from build123d import *

# Parameters (mm, degrees)
F0_W     = 3
F0_H     = 3
F1_DEPTH = 0.15
F2_DEPTH = 1.9
F3_W     = 0.15
F3_H     = 7
F4_DEPTH = 5
F6_DEPTH = 25
F7_R     = 0.5


with BuildPart() as f1:
    # F0 (on Top) → F1 (new body)
    with BuildSketch(Plane.XY):
        with Locations((72.2, 2)):
            Rectangle(F0_W, F0_H)
        with BuildLine():
            Line((10.1, -0.5), (10.1, -3.5))
            Line((10.1, -3.5), (20.2, -3.5))
            Line((20.2, -3.5), (30.3, -3.5))
            Line((30.3, -3.5), (30.3, -0.5))
            Line((30.3, -0.5), (25.7, -0.5))
            ThreePointArc((25.7, -0.5), (25.4171572875, -0.3828427125), (25.3, -0.1))
            Line((25.3, -0.1), (25.3, 0.1))
            ThreePointArc((25.3, 0.1), (25.4171572875, 0.3828427125), (25.7, 0.5))
            Line((25.7, 0.5), (30.3, 0.5))
            Line((30.3, 0.5), (30.3, 3.5))
            Line((30.3, 3.5), (20.2, 3.5))
            Line((20.2, 3.5), (10.1, 3.5))
            Line((10.1, 3.5), (10.1, 0.5))
            Line((10.1, 0.5), (14.7, 0.5))
            ThreePointArc((14.7, 0.5), (14.9828427125, 0.3828427125), (15.1, 0.1))
            Line((15.1, 0.1), (15.1, -0.1))
            ThreePointArc((15.1, -0.1), (14.9828427125, -0.3828427125), (14.7, -0.5))
            Line((14.7, -0.5), (10.1, -0.5))
        make_face()
        with BuildLine():
            Line((30.3, -0.5), (30.3, -3.5))
            Line((30.3, -3.5), (40.4, -3.5))
            Line((40.4, -3.5), (50.5, -3.5))
            Line((50.5, -3.5), (50.5, -0.5))
            Line((50.5, -0.5), (45.9, -0.5))
            ThreePointArc((45.9, -0.5), (45.6171572875, -0.3828427125), (45.5, -0.1))
            Line((45.5, -0.1), (45.5, 0.1))
            ThreePointArc((45.5, 0.1), (45.6171572875, 0.3828427125), (45.9, 0.5))
            Line((45.9, 0.5), (50.5, 0.5))
            Line((50.5, 0.5), (50.5, 3.5))
            Line((50.5, 3.5), (40.4, 3.5))
            Line((40.4, 3.5), (30.3, 3.5))
            Line((30.3, 3.5), (30.3, 0.5))
            Line((30.3, 0.5), (34.9, 0.5))
            ThreePointArc((34.9, 0.5), (35.1828427125, 0.3828427125), (35.3, 0.1))
            Line((35.3, 0.1), (35.3, -0.1))
            ThreePointArc((35.3, -0.1), (35.1828427125, -0.3828427125), (34.9, -0.5))
            Line((34.9, -0.5), (30.3, -0.5))
        make_face()
        with BuildLine():
            Line((50.5, -0.5), (50.5, -3.5))
            Line((50.5, -3.5), (60.6, -3.5))
            Line((60.6, -3.5), (70.7, -3.5))
            Line((70.7, -3.5), (70.7, -0.5))
            Line((70.7, -0.5), (66.1, -0.5))
            ThreePointArc((66.1, -0.5), (65.8171572875, -0.3828427125), (65.7, -0.1))
            Line((65.7, -0.1), (65.7, 0.1))
            ThreePointArc((65.7, 0.1), (65.8171572875, 0.3828427125), (66.1, 0.5))
            Line((66.1, 0.5), (70.7, 0.5))
            Line((70.7, 0.5), (70.7, 3.5))
            Line((70.7, 3.5), (60.6, 3.5))
            Line((60.6, 3.5), (50.5, 3.5))
            Line((50.5, 3.5), (50.5, 0.5))
            Line((50.5, 0.5), (55.1, 0.5))
            ThreePointArc((55.1, 0.5), (55.3828427125, 0.3828427125), (55.5, 0.1))
            Line((55.5, 0.1), (55.5, -0.1))
            ThreePointArc((55.5, -0.1), (55.3828427125, -0.3828427125), (55.1, -0.5))
            Line((55.1, -0.5), (50.5, -0.5))
        make_face()
        with BuildLine():
            Line((0, 3.5), (0, -3.5))
            Line((0, -3.5), (10.1, -3.5))
            Line((10.1, -3.5), (10.1, -0.5))
            Line((10.1, -0.5), (5.5, -0.5))
            ThreePointArc((5.5, -0.5), (5.2171572875, -0.3828427125), (5.1, -0.1))
            Line((5.1, -0.1), (5.1, 0.1))
            ThreePointArc((5.1, 0.1), (5.2171572875, 0.3828427125), (5.5, 0.5))
            Line((5.5, 0.5), (10.1, 0.5))
            Line((10.1, 0.5), (10.1, 3.5))
            Line((10.1, 3.5), (0, 3.5))
        make_face()
        with Locations((72.2, -2)):
            Rectangle(F0_W, F0_H)
    extrude(amount=F1_DEPTH)

    # F2 (add): a face of the model
    f2_faces = [f1.faces().sort_by_distance(p)[0] for p in [
        (0, 0, 0.075),
    ]]
    extrude(f2_faces, amount=F2_DEPTH)

    # F3 (on face) → F4 (join)
    with BuildSketch(Plane(origin=(0, 0, 0), x_dir=(1, 0, 0), z_dir=(0, 0, -1))):
        with Locations((-1.825, 0)):
            Rectangle(F3_W, F3_H)
    extrude(amount=F4_DEPTH)

    # F5 (on face) → F6 (cut)
    with BuildSketch(Plane(origin=(-1.9, 0, 0), x_dir=(0, -1, 0), z_dir=(-1, 0, 0))):
        with BuildLine():
            ThreePointArc((0.5, -3.75), (0.3828427125, -3.4671572875), (0.1, -3.35))
            Line((0.1, -3.35), (-0.1, -3.35))
            ThreePointArc((-0.1, -3.35), (-0.3828427125, -3.4671572875), (-0.5, -3.75))
            Line((-0.5, -3.75), (-0.5, -5))
            Line((-0.5, -5), (0.5, -5))
            Line((0.5, -5), (0.5, -3.75))
        make_face()
    extrude(amount=-F6_DEPTH, mode=Mode.SUBTRACT)

    # F7
    f7_edges = [f1.edges().sort_by_distance(p)[0] for p in [
        (-1.9, 0, 0.15),
        (-1.75, 0, 0),
    ]]
    fillet(f7_edges, radius=F7_R)


solid = f1.part
Source: CAD feature listing. Evaluate the final solid. Frame: model axes, mm. Round coordinates to 2 decimals unless told otherwise and drop trailing zeros. Loops run counter-clockwise (first coordinate to the right, second up) from the corner with the lowest first, then second, coordinate; pieces in that order, holes last. Notation, with made-up numbers: M 36,89.25 L 57,89.25 A17 cw 57,93.25 Z; hole C 32.5,-28.75 d2. An arc over 180 degrees is marked long. Answer as CSV lines item,"result".
Q1. Cut plane B-B (y = -1.25). Return the cut outline in (x, z), plus the area to 3 significant figures.
Verdict:
outline,"M -1.9,-5 L -1.75,-5 L -1.75,-0.5 A0.5 cw -1.25,0 L 73.7,0 L 73.7,0.15 L -1.4,0.15 A0.5 ccw -1.9,-0.35 Z"
area,"12.1 mm^2"
Q2. Cut plane C-C (z = -2.3). Return the cut outline in (x, y).
Verdict:
outline,"M -1.9,-3.5 L -1.75,-3.5 L -1.75,3.5 L -1.9,3.5 Z"
Q3. Cut plane A-A (x = 12). Return the cut outline in (y, z).
Verdict:
outline,"M -3.5,0 L -0.5,0 L -0.5,0.15 L -3.5,0.15 Z; M 0.5,0 L 3.5,0 L 3.5,0.15 L 0.5,0.15 Z"
Q4. Contact query for flat-ended pins moving along their axis: pin 1 (2 mm diameter, centred on x = 40, y = 0, fed in from -Z); pin 2 (2 mm diameter, centred on y = -0.5, z = -4, fed in from +X). Output: stop coordinate, or through.
Verdict:
pin 1,"stops at z = 0"
pin 2,"stops at x = -1.75"
Q5. Cut plane D-D (x = 3). Return the cut outline in (y, z).
Verdict:
outline,"M -3.5,0 L 3.5,0 L 3.5,0.15 L -3.5,0.15 Z"
Q6. Line query: line 1 along Z through (x, y) = (52, -0.75); line 2 along X through (y, z) = (1.5, -0.4); line 3 along X through (y, z) = (1.75, -0.2). Output: solid intervals per line, ascending.
Verdict:
line 1,"z = 0 to 0.15"
line 2,"x = -1.9 to -1.74"
line 3,"x = -1.88 to -1.65"
